Could you check a few things on this model? Use its own coordinates, in mm. A direction names the side the tool comes from. Give positions to 0.01 mm unless a question says otherwise; leave off trailing zeros. Order: outer loops, then holes, each group sorted by start corner. A loop starts at its lowest first (then second) coordinate and runs counter-clockwise, first axis right, second up. Notation, with made-up numbers: (66, -30) -> (75, -30) arc R19 ccw to (75, -3) -> close; hole circle Ø8 at (12, 17.5). An arc over 180 degrees is marked (long way). One line per item, written item: value.
```python
from build123d import *

# Parameters (mm, degrees)
BOSS_EXTRUDE1_DEPTH = 5
SKETCH5_R           = 1.25
CUT_EXTRUDE1_DEPTH  = 3.5


with BuildPart() as part:
    # Sketch1 → Boss-Extrude1 (new body)
    with BuildSketch(Plane(origin=(0, 0, 0), x_dir=(1, 0, 0), z_dir=(0, 1, 0))):
        with BuildLine():
            Line((-2.5, -30.899029111), (-2.5, -24.874685928))
            ThreePointArc((-2.5, -24.874685928), (-25, 0), (-2.5, 24.874685928))
            Line((-2.5, 24.874685928), (-2.5, 30.899029111))
            ThreePointArc((-2.5, 30.899029111), (-31, 0), (-2.5, -30.899029111))
        make_face()
        with BuildLine():
            Line((0, -31), (0, -25))
            ThreePointArc((0, -25), (-1.251569376, -24.968651828), (-2.5, -24.874685928))
            Line((-2.5, -24.874685928), (-2.5, -30.899029111))
            ThreePointArc((-2.5, -30.899029111), (-1.251019097, -30.974746992), (0, -31))
        make_face()
        with BuildLine():
            Line((0, -40), (0, -31))
            ThreePointArc((0, -31), (-1.251019097, -30.974746992), (-2.5, -30.899029111))
            Line((-2.5, -30.899029111), (-2.5, -40))
            Line((-2.5, -40), (0, -40))
        make_face()
        with BuildLine():
            Line((-2.5, 30.899029111), (-2.5, 24.874685928))
            ThreePointArc((-2.5, 24.874685928), (-1.251569376, 24.968651828), (0, 25))
            Line((0, 25), (0, 31))
            ThreePointArc((0, 31), (-1.251019097, 30.974746992), (-2.5, 30.899029111))
        make_face()
        with BuildLine():
            Line((-2.5, 40), (-2.5, 30.899029111))
            ThreePointArc((-2.5, 30.899029111), (-1.251019097, 30.974746992), (0, 31))
            Line((0, 31), (0, 40))
            Line((0, 40), (-2.5, 40))
        make_face()
    extrude(amount=BOSS_EXTRUDE1_DEPTH)

    # Sketch5 → Cut-Extrude1 (cut, through all)
    with BuildSketch(Plane.ZY.offset(2.5)):
        with Locations((-35.899029111, 2.5)):
            Circle(SKETCH5_R)
        with Locations((35.899029111, 2.5)):
            Circle(SKETCH5_R)
    extrude(amount=-CUT_EXTRUDE1_DEPTH, mode=Mode.SUBTRACT)


solid = part.part
```
1) Suppose I cut it at A-A, the plane y = 2.5. Write out the boundary of the cut face in (x, z), then the cut area to 3 significant figures.
Answer below:
outline: (-2.5, -40) -> (0, -40) -> (0, -37.15) -> (-2.5, -37.15) -> close; (-2.5, -34.65) -> (0, -34.65) -> (0, -25) arc R25 cw to (0, 25) -> (0, 34.65) -> (-2.5, 34.65) -> (-2.5, 30.9) arc R31 ccw to (-2.5, -30.9) -> close; (-2.5, 37.15) -> (0, 37.15) -> (0, 40) -> (-2.5, 40) -> close
area: 560 mm2
2) Suppose I cut it at D-D, the plane x = -23. Write out the boundary of the cut face in (y, z), then the cut area to 3 significant figures.
Answer below:
outline: (0, -20.78) -> (5, -20.78) -> (5, -9.8) -> (0, -9.8) -> close; (0, 9.8) -> (5, 9.8) -> (5, 20.78) -> (0, 20.78) -> close
area: 110 mm2
3) We'd pull the mould along Y, two halves only. Please class faces 1 (the cylindrical face through (-1.27, 2.55, 34.65)), 2 (the flat face through (-26, 5, 0)), 3 (the flat face through (0, 2, -32)): +Y half, -Y half, draft (parallel to the pull), parting line (faces both ways), or undercut.
Answer below:
face 1: undercut
face 2: +Y half
face 3: draft
4) For P1, Ø1.5, axis at y = 1.5, z = -10.5, coming from the +X side; P2, Ø3, axis at y = 2.5, z = 35.9, coming from the -X side, each with a flat end and sliding along its axis, tell me the tip position at first contact or that it passes through.
Answer below:
P1: stops at x = -22.33
P2: stops at x = -2.5
5) If I drill on line 1 along Z through (x, y) = (-18, 4.2); line 2 along X through (y, z) = (1.9, 31); line 3 along Z through (x, y) = (-18.5, 4.55), over which ranges is the centre line in solid material (lowest first)?
Answer below:
line 1: z = -25.24 to -17.35, 17.35 to 25.24
line 2: x = -2.5 to 0
line 3: z = -24.87 to -16.82, 16.82 to 24.87
6) For faces 4 (the flat face through (-2.5, 2, 34)), 5 (the cylindrical face through (-30.993, 2.465, -0.647)), 6 (the flat face through (-2.5, 1.9, -34.5)), which set-ups out of +Z, -Z, +X, -X, +Y, -Y let a thin tool reach every point of the face, with its end or its side?
Answer below:
face 4: +Z, -X, +Y, -Y
face 5: -X, +Y, -Y
face 6: -Z, -X, +Y, -Y
7) Suppose I cut it at B-B, the plane x = -12.5. Write out the boundary of the cut face in (y, z), then the cut area to 3 significant figures.
Answer below:
outline: (0, -28.37) -> (5, -28.37) -> (5, -21.65) -> (0, -21.65) -> close; (0, 21.65) -> (5, 21.65) -> (5, 28.37) -> (0, 28.37) -> close
area: 67.2 mm2
8) Suppose I cut it at C-C, the plane z = 33.5. Write out the boundary of the cut face in (x, y).
Answer below:
outline: (-2.5, 0) -> (0, 0) -> (0, 5) -> (-2.5, 5) -> close
